Autodesk Inventor part; units mm, degrees
ref_plane "YZ Plane" through (0, 0, 0) normal (1, 0, 0) x (0, 1, 0)
ref_plane "XZ Plane" through (0, 0, 0) normal (0, 1, 0) x (-1, 0, 0)
ref_plane "XY Plane" through (0, 0, 0) normal (0, 0, 1) x (1, 0, 0)
sketch "Эскиз1" plane through (0, 0, 0) normal (0, 1, 0) x (-1, 0, 0)
  circle A0 centre (-168.9344, 188.7011) radius 75 construction
  circle A1 centre (-108.2116, 232.7209) radius 3.05
  circle A2 centre (-192.0353, 260.0548) radius 3.05
  circle A3 centre (-243.9343, 188.7803) radius 3.05
  circle A4 centre (-192.186, 117.3964) radius 3.05
  circle A5 centre (-108.3047, 144.5532) radius 3.05
  arc A6 (-148.9344, 111.2415) -> (-188.9344, 111.2415) centre (-168.9344, 188.7011) ccw
  line L0 (-188.9344, 88.7011) -> (-148.9344, 88.7011)
  line L1 (-148.9344, 88.7011) -> (-148.9344, 111.2415)
  line L2 (-188.9344, 111.2415) -> (-188.9344, 88.7011)
  circle A7 centre (-168.9344, 188.7011) radius 10
  point P0 (0, 0)
  dimension "d4" = 150
  dimension "d5" = 6.1
  dimension "d8" = 360
  dimension "d10" = 160
  dimension "d13" = 20
  dimension "d14" = 40
  dimension "d15" = 100
  dimension "d16" = 20
extrude "Выдавливание1" add sketch "Эскиз1" along normal blind 3
equation "\"d5\" = d_main_screw_holes"
equation "\"d14\" = hight_coxa"
equation "\"d16\" = d_main_shaft"
equation "\"d2\" = thickness_steel"
equation "\"tolerance_plazma\" = 0.1"
equation "\"thickness_steel\" = 3"
equation "\"d_main_screw_holes\" = 6.1"
equation "\"d_main_shaft\" = 20"
equation "\"thickness_profile_tibea\" = 3"
equation "\"hight_shaft_shift\" = 37"
equation "\"thickness_profile_femur\" = 3"
equation "\"width_shaft_shift\" = 35"
equation "\"width_flattened_surface\" = 12"
equation "\"length_coxa\" = 100"
equation "\"hight_coxa\" = 40"
properties part number "femur_motor_steel" material "Сталь"
The listing builds one solid part. Answer for the finished solid, in the listing's coordinates (mm). Give positions to 0.01 mm unless a question says otherwise; leave off trailing zeros. Write each loop counter-clockwise with the first axis right and the second up, starting at its lowest first coordinate (ties: lowest second). Pieces come first, ordered by that corner, then holes.
1) Section C-C (x = 170) is taken. Write down the section's boundary in (y, z).
2) Given P1, Ø0.9, axis at y = 1, z = 95.5, coming from the +X side, flat-ended and moving along its own axis, determine where the tip first touches the part or whether it passes through.
3) Section B-B (z = 182.5) is taken. Write down the section's boundary in (x, y).
4) Find the intervals of material crossed by L1, parallel to X at y = 0.95, z = 188.5; L2, parallel to Z at x = 106, y = 2.95; L3, parallel to Z at x = 107, y = 0.9, in increasing order.
5) Section D-D (z = 106.5) is taken. Write down the section's boundary in (x, y), and give its area (3 significant figures).
6) Section A-A (y = 0.5) is taken. Write down the section's boundary in (x, z), and give its area (3 significant figures).
7) For a pull along X with two mould halves and no side action, classify faces 1 (the face through (106.804, 1.479, 235.427)), 2 (the face through (172.169, 1.479, 268.636)), 3 (the face through (170, 3, 200)) as pulls with the +X half, pulls with the -X half, needs draft (parallel to the pull), parting line crosses it, or undercut.
Response:
1. outline: (0, 88.7) - (3, 88.7) - (3, 178.76) - (0, 178.76) - close; (0, 198.64) - (3, 198.64) - (3, 268.69) - (0, 268.69) - close
2. P1: stops at x = 188.93
3. outline: (89.18, 0) - (161.09, 0) - (161.09, 3) - (89.18, 3) - close; (176.78, 0) - (248.69, 0) - (248.69, 3) - (176.78, 3) - close
4. L1: x = 88.93 to 158.94, 178.93 to 240.9, 246.97 to 248.93
4. L2: z = 139.31 to 142.56, 146.55 to 230.62, 234.82 to 238.09
4. L3: z = 138.06 to 141.8, 147.31 to 229.92, 235.52 to 239.34
5. outline: (148.93, 0) - (188.93, 0) - (188.93, 3) - (148.93, 3) - close
5. area: 120 mm2
6. outline: (148.93, 88.7) - (188.93, 88.7) - (188.93, 111.24) arc R80 ccw (long way) to (148.93, 111.24) - close; hole circle Ø6.1 at (108.21, 232.72); hole circle Ø6.1 at (108.3, 144.55); hole circle Ø20 at (168.93, 188.7); hole circle Ø6.1 at (192.04, 260.05); hole circle Ø6.1 at (192.19, 117.4); hole circle Ø6.1 at (243.93, 188.78)
6. area: 20,500 mm2
7. face 1: undercut
7. face 2: parting line crosses it
7. face 3: needs draft
